from build123d import *

# Parameters (mm, degrees)
SKETCH1_R               = 0.79375
BOSS_EXTRUDE1_DEPTH     = 2.9718
SKETCH2_W               = 8.560637789
SKETCH2_H               = 1.27
CUT_EXTRUDE1_DEPTH      = 9.983262208
CUT_EXTRUDE1_DEPTH_BACK = 3.38125
SKETCH1_4_R             = 0.508
CUT_EXTRUDE3_DEPTH      = 3.9718
CUT_EXTRUDE3_DEPTH_BACK = 1


with BuildPart() as part:
    # Sketch1 → Boss-Extrude1 (new body)
    with BuildSketch(Plane.XY):
        with BuildLine():
            Line((-38.58806132, -2.249205074), (-19.977544146, 4.220762208))
            Line((-19.977544146, 4.220762208), (-0.641288821, -1.994960876))
            ThreePointArc((-0.641288821, -1.994960876), (1.989850963, -0.656972903), (0.672616276, 1.984617745))
            Line((0.672616276, 1.984617745), (-19.977544146, 8.983262208))
            Line((-19.977544146, 8.983262208), (-40.123930756, 2.258747435))
            ThreePointArc((-40.123930756, 2.258747435), (-41.624019757, -0.76794954), (-38.58806132, -2.249205074))
        make_face()
        with Locations((-39.37, 0)):
            Circle(SKETCH1_R, mode=Mode.SUBTRACT)
    extrude(amount=BOSS_EXTRUDE1_DEPTH)

    # Sketch2 → Cut-Extrude1 (cut, two sides)
    with BuildSketch(Plane(origin=(0, 0, 0), x_dir=(1, 0, 0), z_dir=(0, 1, 0))) as cut_extrude1_sk:
        with Locations((0.025818894, -1.4859)):
            Rectangle(SKETCH2_W, SKETCH2_H)
    extrude(amount=CUT_EXTRUDE1_DEPTH, mode=Mode.SUBTRACT)
    extrude(cut_extrude1_sk.sketch, amount=-CUT_EXTRUDE1_DEPTH_BACK, mode=Mode.SUBTRACT)

    # Sketch1<4> → Cut-Extrude3 (cut, two sides)
    with BuildSketch(Plane.XY) as cut_extrude3_sk:
        Circle(SKETCH1_4_R)
    extrude(amount=CUT_EXTRUDE3_DEPTH, mode=Mode.SUBTRACT)
    extrude(cut_extrude3_sk.sketch, amount=-CUT_EXTRUDE3_DEPTH_BACK, mode=Mode.SUBTRACT)


solid = part.part
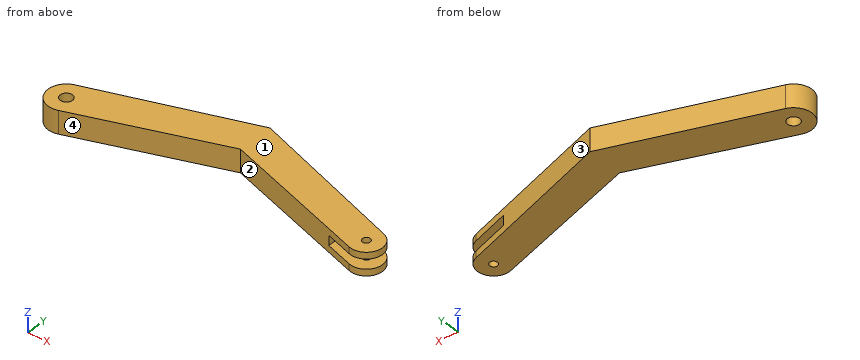
Input: part model. Units: mm. Frame: model coordinates. Face numbers are marked on the shaded views. Give positions to 0.01 mm unless a question says otherwise; leave off trailing zeros. Loops run counter-clockwise (first coordinate to the right, second up) from the corner with the lowest first, then second, coordinate; pieces in that order, holes last. Notation, with made-up numbers: M 13.5,43.5 L 48.5,43.5 A18 ccw 48.5,47.5 Z; hole C 56.5,35.25 d2. An arc over 180 degrees is marked long. Use one line per item in the form item = value.
1. Section query D-D, the plane x = 0. Return the cut outline in (y, z).
Numbers:
outline = M -2.1,0 L -0.51,0 L -0.51,0.85 L -2.1,0.85 Z; M -2.1,2.12 L -0.51,2.12 L -0.51,2.97 L -2.1,2.97 Z; M 0.51,0 L 2.21,0 L 2.21,0.85 L 0.51,0.85 Z; M 0.51,2.12 L 2.21,2.12 L 2.21,2.97 L 0.51,2.97 Z
2. Section query B-B, the plane z = 1.75. Return the cut outline in (x, y), and give its area (3 significant figures).
Numbers:
outline = M -40.12,2.26 A2.38 ccw long -38.59,-2.25 L -19.98,4.22 L -4.25,-0.83 L -4.25,3.65 L -19.98,8.98 Z; hole C -39.37,0 d1.59
area = 175 mm²
3. Pull-direction query (X, two-part tool) for the marked faces 1, 2, 3 and 4; classes: released by +X, released by -X, zero draft, split by the parting line, or undercut.
Numbers:
face_1 = zero draft
face_2 = undercut
face_3 = released by +X
face_4 = undercut
4. Section query C-C, the plane x = -39.37. Return the cut outline in (y, z), and give its area (3 significant figures).
Numbers:
outline = M -2.38,0 L -0.79,0 L -0.79,2.97 L -2.38,2.97 Z; M 0.79,0 L 2.51,0 L 2.51,2.97 L 0.79,2.97 Z
area = 9.82 mm²
5. Line query: L1, parallel to Y at x = -39, z = 1.95; L2, parallel to Y at x = 0, z = 2.4; L3, parallel to Y at x = -28.5, z = 2.8. Output: solid intervals per line, ascending.
Numbers:
L1 = -2.35 to -0.7, 0.7 to 2.63
L2 = -2.1 to -0.51, 0.51 to 2.21
L3 = 1.26 to 6.14
6. First-contact query: pin 1 (1.5 mm diameter, centred on x = -18, z = 0.5, fed in from +Y). Flat tip, straight axial feed; report the tip coordinate or a pass-through.
Numbers:
pin_1 = 8.57
7. Section query A-A, the plane y = 0. Return the cut outline in (x, z).
Numbers:
outline = M -41.75,0 L -40.16,0 L -40.16,2.97 L -41.75,2.97 Z; M -38.58,0 L -32.12,0 L -32.12,2.97 L -38.58,2.97 Z; M -6.85,0 L -0.51,0 L -0.51,0.85 L -4.25,0.85 L -4.25,2.12 L -0.51,2.12 L -0.51,2.97 L -6.85,2.97 Z; M 0.51,0 L 2.1,0 L 2.1,0.85 L 0.51,0.85 Z; M 0.51,2.12 L 2.1,2.12 L 2.1,2.97 L 0.51,2.97 Z
